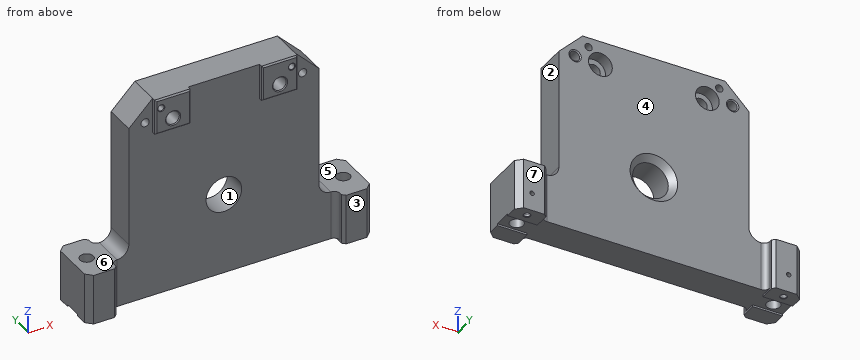
```python
from build123d import *

# Parameters (mm, degrees)
SKETCH1_W                                     = 152.4
SKETCH1_H                                     = 16.51
EXTRUDE1_DEPTH                                = 11.1252
SKETCH2_W                                     = 101.6
SKETCH2_H                                     = 16.51
EXTRUDE2_DEPTH                                = 99.3648
SKETCH4_W                                     = 19.05
SKETCH4_H                                     = 19.05
EXTRUDE4_DEPTH                                = 2.54
SKETCH23_W                                    = 25.4
SKETCH23_H                                    = 15.8877
EXTRUDE17_DEPTH                               = 16.51
SKETCH45_W                                    = 15.875
SKETCH45_H                                    = 6.0325
EXTRUDE20_DEPTH                               = 27.0129
EXTRUDE21_DEPTH                               = 1.016
FILLET3_R                                     = 3.175
F_1_4_CLEARANCE_HOLE1_D                       = 7.14248
CBORE_FOR_SOCKET_HEAD_CAP_SCREW0_AT_2_COUNT   = 2
CBORE_FOR_SOCKET_HEAD_CAP_SCREW0_AT_2_PITCH   = 57.15
F_1_8_PRESS_PIN_HOLES_AT_2_COUNT              = 2
F_1_8_PRESS_PIN_HOLES_AT_2_PITCH              = 137.16
F_3_32_0_09375_DIAMETER_HOLE1_D               = 2.38125
F_3_32_0_09375_DIAMETER_HOLE1_DEPTH           = 12.7
F_3_32_0_09375_DIAMETER_HOLE1_TIP             = 0.715399675
F_3_32_0_09375_DIAMETER_HOLE2_D               = 2.38125
F_3_32_0_09375_DIAMETER_HOLE2_DEPTH           = 4.191
F_3_32_0_09375_DIAMETER_HOLE2_TIP             = 0.715399675
FILLET4_R                                     = 6.35
CHAMFER6_SIZE                                 = 3.175
CHAMFER7_SIZE                                 = 12.7
CHAMFER8_SIZE                                 = 1.5875
CHAMFER9_SIZE                                 = 0.762
CBORE_FOR_6_SOCKET_HEAD_CAP_SCREW2_AT_2_COUNT = 2
CBORE_FOR_6_SOCKET_HEAD_CAP_SCREW2_AT_2_PITCH = 69.85
TAPPED_HOLE_FOR_8_32_HELICOIL2_AT_2_COUNT     = 2
TAPPED_HOLE_FOR_8_32_HELICOIL2_AT_2_PITCH     = 84.218409794


with BuildPart() as part:
    # Sketch1 → Extrude1 (new body)
    with BuildSketch(Plane.XY):
        with Locations((0, 36.195)):
            Rectangle(SKETCH1_W, SKETCH1_H)
    extrude(amount=EXTRUDE1_DEPTH)

    # Sketch2 → Extrude2 (add)
    with BuildSketch(Plane.XY.offset(11.1252)):
        with Locations((0, 36.195)):
            Rectangle(SKETCH2_W, SKETCH2_H)
    extrude(amount=EXTRUDE2_DEPTH)

    # Sketch4 → Extrude4 (add)
    with BuildSketch(Plane.XZ.offset(-27.94)):
        with Locations((-28.575, 100.965)):
            Rectangle(SKETCH4_W, SKETCH4_H)
        with Locations((28.575, 100.965)):
            Rectangle(SKETCH4_W, SKETCH4_H)
    extrude(amount=EXTRUDE4_DEPTH)

    # Sketch23 → Extrude17 (add)
    with BuildSketch(Plane(origin=(0, 44.45, 0), x_dir=(1, 0, 0), z_dir=(0, 1, 0))):
        with Locations((63.5, -19.06905)):
            Rectangle(SKETCH23_W, SKETCH23_H)
        with Locations((-63.5, -19.06905)):
            Rectangle(SKETCH23_W, SKETCH23_H)
    extrude(amount=-EXTRUDE17_DEPTH)

    # Sketch45 → Extrude20 (add)
    with BuildSketch(Plane(origin=(0, 0, 0), x_dir=(-1, 0, 0), z_dir=(0, 0, -1))):
        with Locations((-68.2625, 47.46625)):
            Rectangle(SKETCH45_W, SKETCH45_H)
        with Locations((-68.2625, 24.92375)):
            Rectangle(SKETCH45_W, SKETCH45_H)
        with Locations((68.2625, 47.46625)):
            Rectangle(SKETCH45_W, SKETCH45_H)
        with Locations((68.2625, 24.92375)):
            Rectangle(SKETCH45_W, SKETCH45_H)
    extrude(amount=-EXTRUDE20_DEPTH)

    # Sketch46 → Extrude21 (cut)
    with BuildSketch(Plane(origin=(0, 0, 0), x_dir=(-1, 0, 0), z_dir=(0, 0, -1))):
        Polygon((-60.325, 44.45), (60.325, 44.45), (60.325, 40.9575), (76.2, 40.9575), (76.2, 31.4325), (60.325, 31.4325), (60.325, 27.94), (-60.325, 27.94), (-60.325, 31.4325), (-76.2, 31.4325), (-76.2, 40.9575), (-60.325, 40.9575), align=None)
    extrude(amount=-EXTRUDE21_DEPTH, mode=Mode.SUBTRACT)

    # Fillet3
    fillet3_edges = [part.edges().sort_by_distance(p)[0] for p in [
        (-60.325, 44.45, 14.01445),
        (-60.325, 27.94, 14.01445),
        (60.325, 27.94, 14.01445),
        (60.325, 44.45, 14.01445),
    ]]
    fillet(fillet3_edges, radius=FILLET3_R)

    # 1/4 Clearance Hole1 (through all)
    with Locations(Plane(origin=(56.815772276, 10.084895152, 27.0129), x_dir=(1, 0, 0), z_dir=(0, 0, 1))):
        with Locations((-125.395772276, 26.110104848), (11.764227724, 26.110104848)):
            Hole(F_1_4_CLEARANCE_HOLE1_D / 2)

    # Sketch30 → 3/4 (0.75) Diameter Hole1 (revolve, cut)
    with BuildSketch(Plane(origin=(0, 44.45, 44.45), x_dir=(0, 0, 1), z_dir=(1, 0, 0))):
        Polygon((0, 0), (0, 22.5425), (10.16, 22.5425), (9.525, 21.9075), (9.525, 3.175), (12.7, 0), align=None)
    revolve(axis=Axis((0, 50.8, 44.45), (0, -1, 0)), mode=Mode.SUBTRACT)

    # Sketch7 → CBORE for  Socket Head Cap Screw0 (revolve, cut)
    with BuildSketch(Plane(origin=(-28.575, 44.45, 97.79), x_dir=(0, 0, 1), z_dir=(1, 0, 0))):
        Polygon((0, 0), (0, 19.05), (4.064, 19.05), (3.57124, 18.55724), (3.57124, 6.35), (6.35, 6.35), (6.35, 0), align=None)
    cbore_for_socket_head_cap_screw0 = revolve(axis=Axis((-28.575, 50.8, 97.79), (0, -1, 0)), mode=Mode.SUBTRACT)

    # CBORE for  Socket Head Cap Screw0 at 2: CBORE for  Socket Head Cap Screw0 ×2
    with Locations(*[(i * CBORE_FOR_SOCKET_HEAD_CAP_SCREW0_AT_2_PITCH, 0, 0) for i in range(1, CBORE_FOR_SOCKET_HEAD_CAP_SCREW0_AT_2_COUNT)]):
        add(cbore_for_socket_head_cap_screw0, mode=Mode.SUBTRACT)

    # Sketch47 → 1/8" Press Pin Holes (revolve, cut)
    with BuildSketch(Plane(origin=(68.58, 45.72, 0), x_dir=(0, 1, 0), z_dir=(1, 0, 0))):
        Polygon((0, 0), (0, 7.303866233), (1.5875, 6.35), (1.5875, 1.524), (1.6002, 1.524), (1.6002, 0.3048), (1.905, 0), align=None)
    f_1_8_press_pin_holes = revolve(axis=Axis((68.58, 45.72, -6.35), (0, 0, 1)), mode=Mode.SUBTRACT)

    # 1/8" Press Pin Holes at 2: 1/8" Press Pin Holes ×2
    with Locations(*[(-i * F_1_8_PRESS_PIN_HOLES_AT_2_PITCH, 0, 0) for i in range(1, F_1_8_PRESS_PIN_HOLES_AT_2_COUNT)]):
        add(f_1_8_press_pin_holes, mode=Mode.SUBTRACT)

    # 3/32 (0.09375) Diameter Hole1
    with Locations(Plane(origin=(0, 0, 0), x_dir=(-1, 0, 0), z_dir=(0, 0, -1))):
        with Locations((-68.58, 45.72), (68.58, 45.72)):
            Hole(F_3_32_0_09375_DIAMETER_HOLE1_D / 2, depth=F_3_32_0_09375_DIAMETER_HOLE1_DEPTH)
            with Locations((0, 0, -(F_3_32_0_09375_DIAMETER_HOLE1_DEPTH + F_3_32_0_09375_DIAMETER_HOLE1_TIP / 2))):  # 118° drill point
                Cone(0, F_3_32_0_09375_DIAMETER_HOLE1_D / 2, F_3_32_0_09375_DIAMETER_HOLE1_TIP, mode=Mode.SUBTRACT)

    # 3/32 (0.09375) Diameter Hole2
    with Locations(Plane(origin=(0, 50.4825, 0), x_dir=(-1, 0, 0), z_dir=(0, 1, 0))):
        with Locations((-68.58, 9.525), (68.58, 9.525)):
            Hole(F_3_32_0_09375_DIAMETER_HOLE2_D / 2, depth=F_3_32_0_09375_DIAMETER_HOLE2_DEPTH)
            with Locations((0, 0, -(F_3_32_0_09375_DIAMETER_HOLE2_DEPTH + F_3_32_0_09375_DIAMETER_HOLE2_TIP / 2))):  # 118° drill point
                Cone(0, F_3_32_0_09375_DIAMETER_HOLE2_D / 2, F_3_32_0_09375_DIAMETER_HOLE2_TIP, mode=Mode.SUBTRACT)

    # Fillet4
    fillet4_edges = [part.edges().sort_by_distance(p)[0] for p in [
        (50.8, 36.195, 27.0129),
        (-50.8, 36.195, 27.0129),
    ]]
    fillet(fillet4_edges, radius=FILLET4_R)

    # Chamfer6
    chamfer6_edges = [part.edges().sort_by_distance(p)[0] for p in [
        (-76.2, 50.4825, 13.50645),
        (-76.2, 21.9075, 13.50645),
        (76.2, 50.4825, 13.50645),
        (76.2, 21.9075, 13.50645),
    ]]
    chamfer(chamfer6_edges, length=CHAMFER6_SIZE)

    # Chamfer7
    chamfer7_edges = [part.edges().sort_by_distance(p)[0] for p in [
        (50.8, 36.195, 110.49),
        (-50.8, 36.195, 110.49),
    ]]
    chamfer(chamfer7_edges, length=CHAMFER7_SIZE)

    # Chamfer8
    chamfer8_edges = [part.edges().sort_by_distance(p)[0] for p in [
        (-60.325, 50.4825, 13.50645),
        (-60.325, 21.9075, 13.50645),
        (60.325, 50.4825, 13.50645),
        (60.325, 21.9075, 13.50645),
    ]]
    chamfer(chamfer8_edges, length=CHAMFER8_SIZE)

    # Chamfer9
    chamfer9_edges = [part.edges().sort_by_distance(p)[0] for p in [
        (28.575, 25.4, 91.44),
        (38.1, 25.4, 100.965),
        (28.575, 25.4, 110.49),
        (19.05, 25.4, 100.965),
        (-19.05, 25.4, 100.965),
        (-28.575, 25.4, 91.44),
        (-38.1, 25.4, 100.965),
        (-28.575, 25.4, 110.49),
    ]]
    chamfer(chamfer9_edges, length=CHAMFER9_SIZE)

    # Sketch53 → CBORE for #6 Socket Head Cap Screw2 (revolve, cut)
    with BuildSketch(Plane(origin=(-34.925, 44.45, 105.41), x_dir=(0, 0, 1), z_dir=(1, 0, 0))):
        Polygon((0, 0), (0, 19.05), (1.905, 19.05), (1.63195, 18.77695), (1.63195, 12.7), (1.984375, 12.7), (1.984375, 0), align=None)
    cbore_for_6_socket_head_cap_screw2 = revolve(axis=Axis((-34.925, 50.8, 105.41), (0, -1, 0)), mode=Mode.SUBTRACT)

    # CBORE for #6 Socket Head Cap Screw2 at 2: CBORE for #6 Socket Head Cap Screw2 ×2
    with Locations(*[(i * CBORE_FOR_6_SOCKET_HEAD_CAP_SCREW2_AT_2_PITCH, 0, 0) for i in range(1, CBORE_FOR_6_SOCKET_HEAD_CAP_SCREW2_AT_2_COUNT)]):
        add(cbore_for_6_socket_head_cap_screw2, mode=Mode.SUBTRACT)

    # Sketch55 → Tapped Hole for #8-32 Helicoil2 (revolve, cut)
    with BuildSketch(Plane(origin=(-42.109204897, 44.45, 98.225795103), x_dir=(0, 0, 1), z_dir=(1, 0, 0))):
        Polygon((0, 0), (0, 22.5425), (2.1971, 22.5425), (2.1971, 10.3632), (2.63779, 10.3632), (2.63779, 0.383481822), (3.302, 0), align=None)
    tapped_hole_for_8_32_helicoil2 = revolve(axis=Axis((-42.109204897, 50.8, 98.225795103), (0, -1, 0)), mode=Mode.SUBTRACT)

    # Tapped Hole for #8-32 Helicoil2 at 2: Tapped Hole for #8-32 Helicoil2 ×2
    with Locations(*[(i * TAPPED_HOLE_FOR_8_32_HELICOIL2_AT_2_PITCH, 0, 0) for i in range(1, TAPPED_HOLE_FOR_8_32_HELICOIL2_AT_2_COUNT)]):
        add(tapped_hole_for_8_32_helicoil2, mode=Mode.SUBTRACT)


solid = part.part
```
Read the model definition and answer for the solid it produces. Units are mm, in the model's axes. Face numbers are marked on the shaded views. A direction names the side the tool comes from. Coordinates: 2 decimals unless noted, no trailing zeros. Loops run counter-clockwise (first coordinate to the right, second up) from the corner with the lowest first, then second, coordinate; pieces in that order, holes last. Notation, with made-up numbers: (-7, 40) -> (16, 40) arc R11 cw to (16, 61) -> close; hole circle Ø10 at (86.25, 11.25). An arc over 180 degrees is marked (long way). Return JSON: item names as keys, results as strings.
Item 1: Flat-ended cylindrical pins translate along their axes: P1, Ø2.5, axis at x = 68.58, y = 45.72, coming from the -Z side; P2, Ø0.9, axis at x = -32.5, y = 27, coming from the -Z side; P3, Ø2, axis at y = 28, z = 75, coming from the +X side. Find the tip coordinate at first contact, or state that the pin passes through.
Answers:
{"P1": "stops at z = 6.55", "P2": "stops at z = 91.44", "P3": "stops at x = 50.8"}
Item 2: For a pull along X with two mould halves and no side action, classify the marked faces 1, 2, 3 and 4 as +X half, -X half, draft (parallel to the pull), parting line (faces both ways), or undercut.
Answers:
{"face 1": "undercut", "face 2": "+X half", "face 3": "draft", "face 4": "undercut"}
Item 3: Find the intervals of material crossed by probe 1 along X at (y, z) = (39.5, 105.41); probe 2 along X at (y, z) = (45.72, 1.25); probe 3 along Z at (x, y) = (15, 28.75), in increasing order.
Answers:
{"probe 1": "x = -43.18 to -36.91, -32.94 to 32.94, 36.91 to 43.18", "probe 2": "x = -76.2 to -70.18, -66.98 to -59.69, 59.69 to 66.98, 70.18 to 76.2", "probe 3": "z = 1.02 to 110.49"}
Item 4: Find section C-C (z = 89). Determine the outline of the cut face in (x, y).
Answers:
{"outline": "(-50.8, 27.94) -> (50.8, 27.94) -> (50.8, 44.45) -> (-50.8, 44.45) -> close"}
Item 5: Find section D-D (x = 49). Determine the outline of the cut face in (y, z), plus the area to 3 significant figures.
Answers:
{"outline": "(27.94, 1.02) -> (44.45, 1.02) -> (44.45, 99.59) -> (27.94, 99.59) -> close", "area": "1,630 mm2"}
Item 6: For the marked faces 5, 6 and 7, determine the directions among +Z, -Z, +X, -X, +Y, -Y from which every point of the face is accessible in a straight line to the end or side of a thin tool.
Answers:
{"face 5": "+Z, +X, +Y, -Y", "face 6": "+Z, -X, +Y, -Y", "face 7": "+Z, -Z, +X, -X, +Y"}
Item 7: Find section B-B (x = 0). Determine the outline of the cut face in (y, z) (3 decimals).
Answers:
{"outline": "(27.94, 1.016) -> (44.45, 1.016) -> (44.45, 31.75) -> (41.275, 34.925) -> (27.94, 34.925) -> close; (27.94, 53.975) -> (41.275, 53.975) -> (44.45, 57.15) -> (44.45, 110.49) -> (27.94, 110.49) -> close"}
Item 8: Find section A-A (z = 44.45). Determine the outline of the cut face in (x, y) (3 decimals).
Answers:
{"outline": "(-50.8, 27.94) -> (-9.525, 27.94) -> (-9.525, 41.275) -> (-12.7, 44.45) -> (-50.8, 44.45) -> close; (9.525, 27.94) -> (50.8, 27.94) -> (50.8, 44.45) -> (12.7, 44.45) -> (9.525, 41.275) -> close"}
